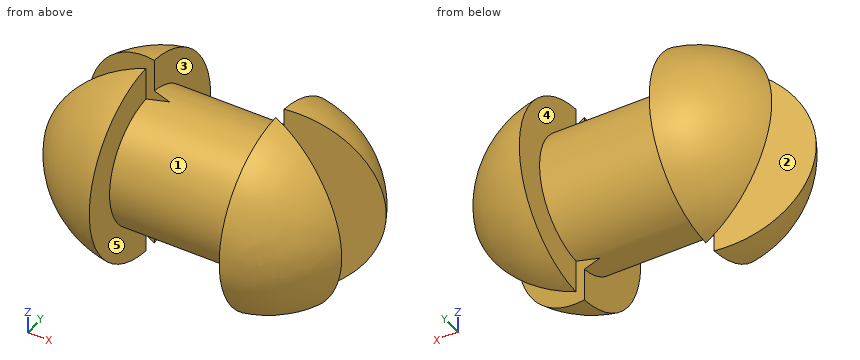
from build123d import *

# Parameters (mm, degrees)
CUT_EXTRUDE1_DEPTH = 20


with BuildPart() as part:
    # Sketch1 → Revolve4 (revolve)
    with BuildSketch(Plane.XY):
        with BuildLine():
            Line((-10, 10), (-10, 15))
            ThreePointArc((-10, 15), (-19.821538313, 9.985820369), (-24.5, 0))
            Line((-24.5, 0), (-7, 0))
            Line((-7, 0), (7, 0))
            Line((7, 0), (24.5, 0))
            ThreePointArc((24.5, 0), (19.821538313, 9.985820369), (10, 15))
            Line((10, 15), (10, 10))
            Line((10, 10), (-10, 10))
        make_face()
    revolve(axis=Axis((-3.122498999, 0, 0), (1, 0, 0)))

    # Sketch2 → Cut-Extrude1 (cut, symmetric)
    with BuildSketch(Plane.XY):
        Polygon((-25, 0), (-7, 0), (-24.964852936, -6.185794935), align=None)
        Polygon((-24.964852936, 6.185794935), (-25, 0), (-7, 0), align=None)
        Polygon((25, 0), (7, 0), (24.964852936, 6.185794935), align=None)
        Polygon((25, 0), (7, 0), (24.964852936, -6.185794935), align=None)
    extrude(amount=CUT_EXTRUDE1_DEPTH, both=True, mode=Mode.SUBTRACT)


solid = part.part
Could you check a few things on this model? Use its own coordinates, in mm. Face numbers are marked on the shaded views. A direction names the side the tool comes from. Coordinates: 2 decimals unless noted, no trailing zeros. Loops run counter-clockwise (first coordinate to the right, second up) from the corner with the lowest first, then second, coordinate; pieces in that order, holes last.
1. I need wall thicknesses on L1, parallel to X at y = 6.5, z = 8; L2, parallel to Y at x = -17, z = 5.5; L3, parallel to Y at x = 14, z = -11.75. Which ranges of each line are inside material? Lowest first, please.
2. We'd pull the mould along Y, two halves only. Please class the marked faces 1, 2 and 3: released by +Y, released by -Y, zero draft, split by the parting line, or undercut.
3. Imagine slicing it at B-B (z = 11.5). Give the number of separate pieces and of enclosed holes in the cut face, and give its area (3 significant figures).
4. Imagine slicing it at A-A (x = 6.5). Please give me the cut outline in (y, z), and give its area (3 significant figures).
5. For P1, Ø3, axis at x = 12, z = -2.5, coming from the +Y side; P2, Ø1.5, axis at x = -0.5, y = 3.5, coming from the -Z side; P3, Ø5, axis at y = 7.5, z = 8, coming from the -X side, each with a flat end and sliding along its axis, tell me the tip position at first contact or that it passes through.
6. For the marked faces 4 and 5, which set-ups out of +Z, -Z, +X, -X, +Y, -Y let a thin tool reach every point of the face, with its end or its side?
Computed values:
1. L1: x = -19.5 to -10, 10 to 19.5
1. L2: y = -11.04 to -3.44, 3.44 to 11.04
1. L3: y = -7.46 to -2.41, 2.41 to 7.46
2. face 1: split by the parting line
2. face 2: undercut
2. face 3: zero draft
3. separate pieces: 4
3. enclosed holes: 0
3. area: 157 mm2
4. outline: circle Ø20 at (0, 0)
4. area: 314 mm2
5. P1: stops at y = 14.78
5. P2: stops at z = -9.61
5. P3: stops at x = -21.13
6. face 4: +Y
6. face 5: -Y
